```python
from build123d import *

# Parameters (mm, degrees)
F1_DEPTH = 6.35
F2_DEPTH = 12.7


with BuildPart() as f1:
    # F0 (on Right) → F1 (new body, symmetric)
    with BuildSketch(Plane.YZ):
        Polygon((0, 0), (0, 254), (-152.4, 254), (-152.4, 50.8), (-330.2, 50.8), (-330.2, 254), (-482.6, 254), (-482.6, 0), (-603.25, 0), (-603.25, -101.6), (-450.85, -101.6), (-387.35, -38.1), (-95.25, -38.1), (-31.75, -101.6), (120.65, -101.6), (120.65, 0), align=None)
    extrude(amount=F1_DEPTH, both=True)

    # F0 (on Right) → F2 (join)
    with BuildSketch(Plane.YZ):
        Polygon((0, 0), (0, 254), (-152.4, 254), (-152.4, 50.8), (-330.2, 50.8), (-330.2, 254), (-482.6, 254), (-482.6, 0), (-603.25, 0), (-603.25, -101.6), (-450.85, -101.6), (-387.35, -38.1), (-95.25, -38.1), (-31.75, -101.6), (120.65, -101.6), (120.65, 0), align=None)
    extrude(amount=F2_DEPTH)


solid = f1.part
```
Read the model definition and answer for the solid it produces. Units are mm, in the model's axes. A direction names the side the tool comes from. Coordinates: 2 decimals unless noted, no trailing zeros. Write each loop counter-clockwise with the first axis right and the second up, starting at its lowest first coordinate (ties: lowest second). Pieces come first, ordered by that corner, then holes. Notation, with made-up numbers: (42, -2.5) - (87, -2.5) arc R20 ccw to (87, 2.5) - close; hole circle Ø4 at (63.25, -10.5). An arc over 180 degrees is marked (long way). Answer as a JSON object with one key per item and string values. Group by question number.
1. A cutting plane is placed at C-C (y = -142). Determine the outline of the cut face in (x, z).
2. The mould has two halves that part along Y. Classify faces 1 (the flat face through (3, -240, 50.8)), 2 (the flat face through (3, 0, 125)), 3 (the flat face through (3, -542, 0)): +Y half, -Y half, draft (parallel to the pull), parting line (faces both ways), or undercut.
3. A cutting plane is placed at B-B (x = 2.75). Determine the outline of the cut face in (y, z), plus the area to 3 significant figures.
4. Consider L1, parallel to Y at x = 12, z = 151.5; L2, parallel to Z at x = 10.25, y = -521.5; L3, parallel to Y at x = 8.5, z = -82. Determine where each line is inside the solid, lowest interval first. Write a range as [from, to].
5. Which of the six approach directions +Z, -Z, +X, -X, +Y, -Y give full straight-line access (tool end or side, diameter ignored) to faces 4 (the flat face through (3, -482.6, 129)), 5 (the flat face through (3.04, -63.94, -69.41)), 6 (the flat face through (3, -152.4, 154)), 7 (the flat face through (3, 61, 0))?
6. A cutting plane is placed at D-D (z = 21.5). Determine the outline of the cut face in (x, y), plus the area to 3 significant figures.
7. Each of these flat-tipped pins is pushed along its axis until it touches: P1, Ø10, axis at x = 0.5, y = -160.5, coming from the +Z side; P2, Ø9.5, axis at x = 0, y = -561.5, coming from the +Z side; P3, Ø1.5, axis at x = 6, z = 53, coming from the -Y side. Where does it stop, or does it pass through?
8. A cutting plane is placed at A-A (z = 102.5). Determine the outline of the cut face in (x, y), plus the area to 3 significant figures.
Worked out:
{
 "1": {"outline": "(-6.35, -38.1) - (12.7, -38.1) - (12.7, 254) - (-6.35, 254) - close"},
 "2": {"face 1": "undercut", "face 2": "+Y half", "face 3": "draft"},
 "3": {"outline": "(-603.25, -101.6) - (-450.85, -101.6) - (-387.35, -38.1) - (-95.25, -38.1) - (-31.75, -101.6) - (120.65, -101.6) - (120.65, 0) - (0, 0) - (0, 254) - (-152.4, 254) - (-152.4, 50.8) - (-330.2, 50.8) - (-330.2, 254) - (-482.6, 254) - (-482.6, 0) - (-603.25, 0) - close", "area": "137,000 mm²"},
 "4": {"L1": "y = [-482.6, -330.2], [-152.4, 0]", "L2": "z = [-101.6, 0]", "L3": "y = [-603.25, -431.25], [-51.35, 120.65]"},
 "5": {"face 4": "+Z, +X, -X, -Y", "face 5": "-Z, +X, -X", "face 6": "+Z, +X, -X", "face 7": "+Z, +X, -X, +Y"},
 "6": {"outline": "(-6.35, -482.6) - (12.7, -482.6) - (12.7, 0) - (-6.35, 0) - close", "area": "9,190 mm²"},
 "7": {"P1": "stops at z = 50.8", "P2": "stops at z = 0", "P3": "stops at y = -482.6"},
 "8": {"outline": "(-6.35, -482.6) - (12.7, -482.6) - (12.7, -330.2) - (-6.35, -330.2) - close; (-6.35, -152.4) - (12.7, -152.4) - (12.7, 0) - (-6.35, 0) - close", "area": "5,810 mm²"}
}
